Verification items for the finished model (mm, model axes). A direction names the side the tool comes from. Give positions to 0.01 mm unless a question says otherwise; leave off trailing zeros. Loops run counter-clockwise (first coordinate to the right, second up) from the corner with the lowest first, then second, coordinate; pieces in that order, holes last. Notation, with made-up numbers: M 20.5,-28 L 41.5,-28 A27 ccw 41.5,2 Z; hole C -34.75,53.5 d7. An arc over 180 degrees is marked long. Use a Markdown table: item, result.
from build123d import *

# Parameters (mm, degrees)
EXTRUDE_1_DEPTH          = 6
CUT_EXTRUDE_1_DEPTH      = 38.363083385
CUT_EXTRUDE_1_DEPTH_BACK = 38.363083385
SKETCH_2_R               = 1.4
SKETCH_3_R               = 4.1
CUT_EXTRUDE_2_DEPTH      = 1.2
SKETCH_4_R               = 4.1
CUT_EXTRUDE_3_DEPTH      = 4
SKETCH_5_R               = 3.5
CUT_EXTRUDE_5_DEPTH      = 38.363083385


with BuildPart() as part:
    # ｽｹｯﾁ1 → ﾎﾞｽ - 押し出し1 (new body)
    with BuildSketch(Plane.XY):
        with BuildLine():
            Line((-0.533333333, 7.982202425), (-30.4, 5.986651819))
            ThreePointArc((-30.4, 5.986651819), (-36, 0), (-30.4, -5.986651819))
            Line((-30.4, -5.986651819), (-0.533333333, -7.982202425))
            ThreePointArc((-0.533333333, -7.982202425), (8, 0), (-0.533333333, 7.982202425))
        make_face()
    extrude(amount=EXTRUDE_1_DEPTH)

    # ｽｹｯﾁ2 → ｶｯﾄ - 押し出し1 (cut, two sides: drawn at the far end of the back side and taken through both)
    with BuildSketch(Plane.XY.offset(-CUT_EXTRUDE_1_DEPTH_BACK)):
        with Locations((-4.242640687, 4.242640687)):
            Circle(SKETCH_2_R)
        with Locations((6, 0)):
            Circle(SKETCH_2_R)
        with Locations((0, 6)):
            Circle(SKETCH_2_R)
        with Locations((-6, 0)):
            Circle(SKETCH_2_R)
        with Locations((-4.242640687, -4.242640687)):
            Circle(SKETCH_2_R)
        with Locations((0, -6)):
            Circle(SKETCH_2_R)
        with Locations((4.242640687, -4.242640687)):
            Circle(SKETCH_2_R)
        with Locations((4.242640687, 4.242640687)):
            Circle(SKETCH_2_R)
    extrude(amount=CUT_EXTRUDE_1_DEPTH + CUT_EXTRUDE_1_DEPTH_BACK, mode=Mode.SUBTRACT)

    # ｽｹｯﾁ3 → ｶｯﾄ - 押し出し2 (cut)
    with BuildSketch(Plane(origin=(0, 0, 0), x_dir=(-1, 0, 0), z_dir=(0, 0, -1))):
        Circle(SKETCH_3_R)
    extrude(amount=-CUT_EXTRUDE_2_DEPTH, mode=Mode.SUBTRACT)

    # ｽｹｯﾁ4 → ｶｯﾄ - 押し出し3 (cut)
    with BuildSketch(Plane.XY.offset(6)):
        with Locations((-30, 0)):
            Circle(SKETCH_4_R)
    extrude(amount=-CUT_EXTRUDE_3_DEPTH, mode=Mode.SUBTRACT)

    # ｽｹｯﾁ5 → ｶｯﾄ - 押し出し5 (cut, through all)
    with BuildSketch(Plane.XY.offset(6)):
        with Locations((-30, 0)):
            Circle(SKETCH_5_R)
    extrude(amount=-CUT_EXTRUDE_5_DEPTH, mode=Mode.SUBTRACT)


solid = part.part
(1) Cross-section at B-B on y = -0.75. Record the cut outline in (x, z).
Results below:
| item | result |
|---|---|
| outline | M -35.95,0 L -33.42,0 L -33.42,2 L -34.03,2 L -34.03,6 L -35.95,6 Z; M -26.58,0 L -7.18,0 L -7.18,6 L -25.97,6 L -25.97,2 L -26.58,2 Z; M -4.82,0 L -4.03,0 L -4.03,1.2 L 4.03,1.2 L 4.03,0 L 4.82,0 L 4.82,6 L -4.82,6 Z; M 7.18,0 L 7.96,0 L 7.96,6 L 7.18,6 Z |
(2) Cross-section at C-C on x = -30. Record the cut outline in (y, z), then the cut area to 3 significant figures.
Results below:
| item | result |
|---|---|
| outline | M -6.01,0 L -3.5,0 L -3.5,2 L -4.1,2 L -4.1,6 L -6.01,6 Z; M 3.5,0 L 6.01,0 L 6.01,6 L 4.1,6 L 4.1,2 L 3.5,2 Z |
| area | 25.4 mm^2 |
(3) Cross-section at D-D on y = -7. Record the cut outline in (x, z), then the cut area to 3 significant figures.
Results below:
| item | result |
|---|---|
| outline | M -15.23,0 L -0.98,0 L -0.98,6 L -15.23,6 Z; M 0.98,0 L 3.87,0 L 3.87,6 L 0.98,6 Z |
| area | 103 mm^2 |
(4) Set-up check for faces 1 (the cylindrical face through (-36, 0, 3)), 2 (the cylindrical face through (0.534, 4.065, 0.592)), 3 (the cylindrical face through (-34.096, 0.18, 4.028)): record each of +Z, -Z, +X, -X, +Y, -Y from which the full face is reachable in a straight line by a thin tool's end or side.
Results below:
| item | result |
|---|---|
| face 1 | +Z, -Z, -X |
| face 2 | -Z |
| face 3 | +Z |
(5) Cross-section at A-A on x = 0. Record the cut outline in (y, z).
Results below:
| item | result |
|---|---|
| outline | M -8,0 L -7.4,0 L -7.4,6 L -8,6 Z; M -4.6,0 L -4.1,0 L -4.1,1.2 L 4.1,1.2 L 4.1,0 L 4.6,0 L 4.6,6 L -4.6,6 Z; M 7.4,0 L 8,0 L 8,6 L 7.4,6 Z |
(6) Draft check along Y on faces 4 (the cylindrical face through (8, 0, 3)), 5 (the flat face through (-14, 0, 0)), 6 (the cylindrical face through (-0.18, 7.39, 2.96)). Enter one of: +Y half, -Y half, draft (parallel to the pull), parting line (faces both ways), or undercut.
Results below:
| item | result |
|---|---|
| face 4 | parting line |
| face 5 | draft |
| face 6 | undercut |
(7) Material ranges on line 1 (X direction, y = 4.75, z = 1.85); line 2 (Y direction, x = -0.5, z = 5.7); line 3 (Y direction, x = -0.5, z = 0.8), recorded low to high.
Results below:
| item | result |
|---|---|
| line 1 | -33.67 to -5.55, -2.94 to -0.63, 0.63 to 2.94, 5.55 to 6.44 |
| line 2 | -7.98 to -7.31, -4.69 to 4.69, 7.31 to 7.98 |
| line 3 | -7.98 to -7.31, -4.69 to -4.07, 4.07 to 4.69, 7.31 to 7.98 |
(8) Gauge pin test, flat ends, axial feed: P1, Ø1.5, axis at x = -14, z = 2, coming from the -Y side; P2, Ø1.7, axis at x = 0, y = 6, coming from the -Z side; P3, Ø1, axis at y = -5.5, z = 1.5, coming from the +X side (3 decimals); P4, Ø3, axis at x = -2, z = 4.5, coming from the -Y side. Record the tip position at first contact, or that the pin passes through.
Results below:
| item | result |
|---|---|
| P1 | y = -7.13 |
| P2 | through |
| P3 | x = 6.245 |
| P4 | y = -7.98 |
